Part model, mm, in its own coordinate system. Face numbers are marked on the shaded views. A direction names the side the tool comes from. Round coordinates to 2 decimals unless told otherwise and drop trailing zeros. Loops run counter-clockwise (first coordinate to the right, second up) from the corner with the lowest first, then second, coordinate; pieces in that order, holes last. Notation, with made-up numbers: (4.5, 16) - (59.5, 16) arc R15 cw to (59.5, 21) - close; hole circle Ø9 at (24.25, 69). An arc over 180 degrees is marked (long way). Write each question's results on one line, items separated by ' | '. Start each with the question number.
(1) Tool access for the marked faces 4, 5, 6 and 7: list every direction of +Z, -Z, +X, -X, +Y, -Y with a clear straight run to the whole face (end or side of a thin tool).
(2) Mould opens along X. For the marked faces 1, 2 and 3 say: released by +X, released by -X, zero draft, split by the parting line, or undercut.
(3) Cut at A-A, the plane z = 10. List the corners of the cut face in (x, y).
(4) Cut at B-B, the plane x = -5. List the corners of the cut face in (y, z), then the cut area to 3 significant figures.
(5) Drill centre lines: L1, parallel to X at y = -59.5, z = 4.6 (3 decimals); L2, parallel to X at y = -61, z = 7.5. Where is each one in solid material? Low to high.
(6) Flat gauge pins, fed straight in: P1, Ø5, axis at y = -59, z = 19, coming from the -X side; P2, Ø5, axis at x = -19.5, y = -58, coming from the +Z side; P3, Ø4, axis at x = 7.5, z = 5.5, coming from the +Y side. Where does each tip first touch, or does it go through?
from build123d import *
from build123d.topology import SkipClean

# Parameters (mm, degrees)
SKETCH2_W             = 4.25
SKETCH2_H             = 10
BOSS_EXTRUDE1_DEPTH   = 32.5
BOSS_EXTRUDE1_2_DEPTH = 32.5
SKETCH3_W             = 28.8
SKETCH3_H             = 10
BOSS_EXTRUDE2_DEPTH   = 3
SKETCH4_W             = 8.25
SKETCH4_H             = 10
SKETCH4_W_2           = 12.5
SKETCH4_W_3           = 4.25
BOSS_EXTRUDE3_DEPTH   = 3
SKETCH5_W             = 2
SKETCH5_H             = 10
BOSS_EXTRUDE4_DEPTH   = 3
CUT_EXTRUDE1_DEPTH    = 3
SKETCH7_W             = 10.25
SKETCH7_H             = 10
SKETCH7_R             = 2.75
BOSS_EXTRUDE5_DEPTH   = 2
FILLET1_R             = 2


with BuildPart() as part:
    # Sketch2 → Boss-Extrude1 (new body)
    with BuildSketch(Plane.XY):
        with Locations((-12.275, -59.5)):
            Rectangle(SKETCH2_W, SKETCH2_H)
    extrude(amount=BOSS_EXTRUDE1_DEPTH)



with BuildPart() as body_2:
    # Sketch2 → Boss-Extrude1 2 (new body)
    with BuildSketch(Plane.XY):
        with Locations((12.275, -59.5)):
            Rectangle(SKETCH2_W, SKETCH2_H)
    extrude(amount=BOSS_EXTRUDE1_2_DEPTH)


with BuildPart() as part_1:
    add(part.part)

    add(body_2.part)  # Boss-Extrude2 merges body 2
    # Sketch3 → Boss-Extrude2 (add)
    with BuildSketch(Plane.XY.offset(32.5)):
        with Locations((0, -59.5)):
            Rectangle(SKETCH3_W, SKETCH3_H)
    extrude(amount=BOSS_EXTRUDE2_DEPTH)

    # Sketch4 → Boss-Extrude3 (add)
    with BuildSketch(Plane(origin=(0, 0, 0), x_dir=(-1, 0, 0), z_dir=(0, 0, -1))):
        with Locations((18.525, -59.5)):
            Rectangle(SKETCH4_W, SKETCH4_H)
        with Locations((-16.4, -59.5)):
            Rectangle(SKETCH4_W_2, SKETCH4_H)
        with Locations((12.275, -59.5)):
            Rectangle(SKETCH4_W_3, SKETCH4_H)
    extrude(amount=-BOSS_EXTRUDE3_DEPTH)

    # Sketch5 → Boss-Extrude4 (add)
    with BuildSketch(Plane(origin=(0, 0, 0), x_dir=(-1, 0, 0), z_dir=(0, 0, -1))):
        with Locations((23.65, -59.5)):
            Rectangle(SKETCH5_W, SKETCH5_H)
        with Locations((-23.65, -59.5)):
            Rectangle(SKETCH5_W, SKETCH5_H)
    extrude(amount=-BOSS_EXTRUDE4_DEPTH)

    # Sketch6 → Cut-Extrude1 (cut)
    with BuildSketch(Plane(origin=(0, 0, 0), x_dir=(-1, 0, 0), z_dir=(0, 0, -1))):
        with BuildLine():
            ThreePointArc((22.275, -59.5), (20.561677147, -56.952883887), (17.556599642, -57.579609407))
            Line((17.556599642, -57.579609407), (21.493400358, -61.420390593))
            ThreePointArc((21.493400358, -61.420390593), (22.072116113, -60.536677147), (22.275, -59.5))
        make_face()
        with BuildLine():
            Line((21.493400358, -61.420390593), (17.556599642, -57.579609407))
            ThreePointArc((17.556599642, -57.579609407), (17.604609407, -61.468400358), (21.493400358, -61.420390593))
        make_face()
        with BuildLine():
            ThreePointArc((-16.775, -59.5), (-16.977883887, -58.463322853), (-17.556599642, -57.579609407))
            Line((-17.556599642, -57.579609407), (-21.493400358, -61.420390593))
            ThreePointArc((-21.493400358, -61.420390593), (-18.488322853, -62.047116113), (-16.775, -59.5))
        make_face()
        with BuildLine():
            Line((-21.493400358, -61.420390593), (-17.556599642, -57.579609407))
            ThreePointArc((-17.556599642, -57.579609407), (-21.445390593, -57.531599642), (-21.493400358, -61.420390593))
        make_face()
    extrude(amount=-CUT_EXTRUDE1_DEPTH, mode=Mode.SUBTRACT)

    # Sketch7 → Boss-Extrude5 (add)
    # profile 1 of 2: a face of its own
    with SkipClean():  # the faces are left unmerged after this step: merging them gives an invalid solid
        with BuildSketch(Plane.XY.offset(3)):
            with Locations((-19.525, -59.5)):
                Rectangle(SKETCH7_W, SKETCH7_H)
            with Locations(Location((-19.525, -59.5, 0), (0, 0, 180))):
                Circle(SKETCH7_R, mode=Mode.SUBTRACT)
        # profile 2 of 2: a face of its own
        with BuildSketch(Plane.XY.offset(3)):
            with Locations((19.525, -59.5)):
                Rectangle(SKETCH7_W, SKETCH7_H)
            with Locations(Location((19.525, -59.5, 0), (0, 0, 180))):
                Circle(SKETCH7_R, mode=Mode.SUBTRACT)
        extrude(amount=BOSS_EXTRUDE5_DEPTH)
    add(part_1.part.scale(1), mode=Mode.REPLACE)  # the faces are merged on a copy

    # Fillet1
    fillet1_edges = [part_1.edges().sort_by_distance(p)[0] for p in [
        (14.4, -59.5, 35.5),
        (-14.4, -59.5, 35.5),
    ]]
    fillet(fillet1_edges, radius=FILLET1_R)


solid = part_1.part
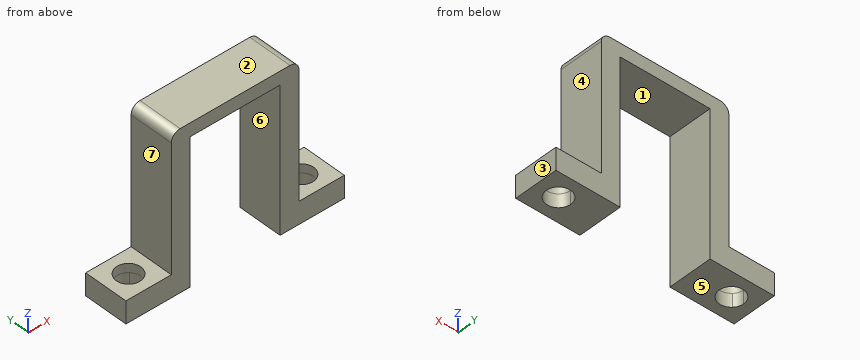
A:
1) face 4: +Z, +X, +Y, -Y | face 5: -Z, +X, -X, +Y, -Y | face 6: -Z, +Y, -Y | face 7: +Z, -X, +Y, -Y
2) face 1: undercut | face 2: zero draft | face 3: released by +X
3) outline: (-14.4, -64.5) - (-10.15, -64.5) - (-10.15, -54.5) - (-14.4, -54.5) - close; (10.15, -64.5) - (14.4, -64.5) - (14.4, -54.5) - (10.15, -54.5) - close
4) outline: (-64.5, 32.5) - (-54.5, 32.5) - (-54.5, 35.5) - (-64.5, 35.5) - close | area: 30.0 mm2
5) L1: -24.65 to -22.275, -16.775 to -10.15, 10.15 to 16.775, 22.275 to 24.65 | L2: -14.4 to -10.15, 10.15 to 14.4
6) P1: x = -14.4 | P2: z = 5 | P3: through
